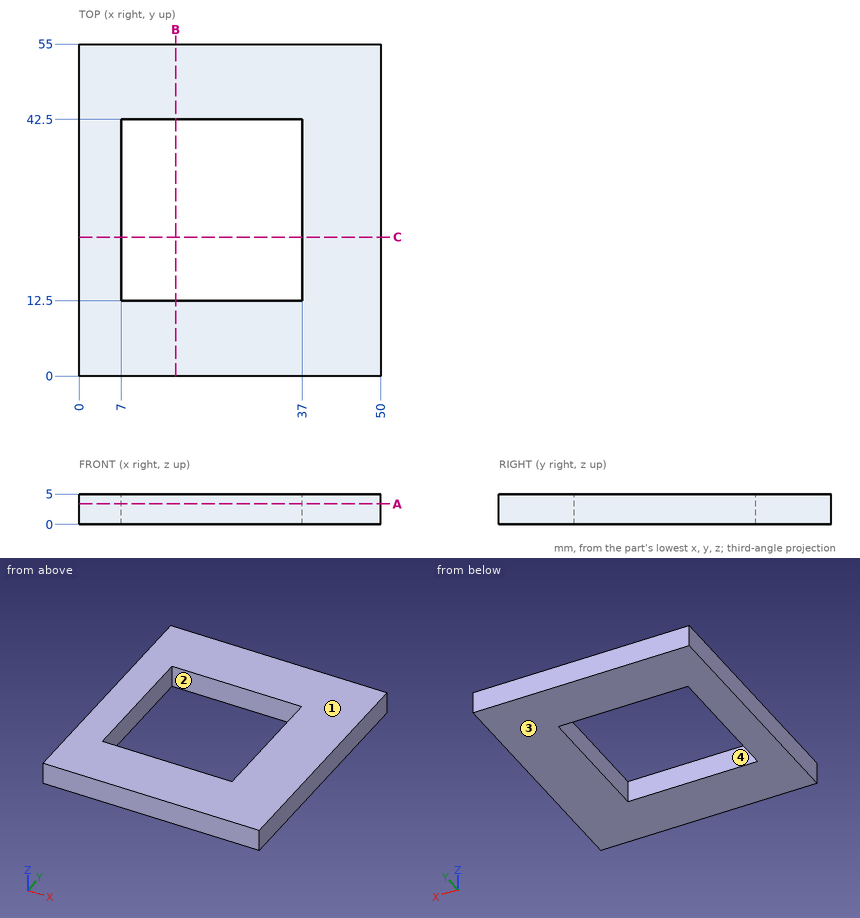
Drawing for the job (mm, zero at the part's lowest x, y, z). A direction names the side the tool comes from. Coordinates: 2 decimals unless noted, no trailing zeros. Order: outer loops, then holes, each group sorted by start corner. A loop starts at its lowest first (then second) coordinate and runs counter-clockwise, first axis right, second up. Notation, with made-up numbers: (17, 89) -> (31, 89) arc R34 cw to (31, 120) -> close; hole circle Ø7 at (-21.75, 23.5). An arc over 180 degrees is marked (long way). One line per item, written item: value.
(1) Slice it at B-B, the plane x = 16. List the corners of the cut face in (y, z), plus the area to 3 significant figures.
Checked values:
outline: (0, 0) -> (12.5, 0) -> (12.5, 5) -> (0, 5) -> close; (42.5, 0) -> (55, 0) -> (55, 5) -> (42.5, 5) -> close
area: 125 mm2
(2) Probe line 1 (X direction, y = 27, z = 0.5); line 2 (Y direction, x = 19.5, z = 2.7). List the from-to ranges inside material, lowest first. Write a range as [from, to].
Checked values:
line 1: [0, 7], [37, 50]
line 2: [0, 12.5], [42.5, 55]
(3) Slice it at A-A, the plane z = 3.4. List the corners of the cut face in (x, y), plus the area to 3 significant figures.
Checked values:
outline: (0, 0) -> (50, 0) -> (50, 55) -> (0, 55) -> close; hole (7, 12.5) -> (37, 12.5) -> (37, 42.5) -> (7, 42.5) -> close
area: 1,850 mm2
(4) Slice it at C-C, the plane y = 23. List the corners of the cut face in (x, z).
Checked values:
outline: (0, 0) -> (7, 0) -> (7, 5) -> (0, 5) -> close; (37, 0) -> (50, 0) -> (50, 5) -> (37, 5) -> close
(5) Mould opens along X. For the marked faces 1 and 2 say: pulls with the +X half, pulls with the -X half, needs draft (parallel to the pull), parting line crosses it, or undercut.
Checked values:
face 1: needs draft
face 2: undercut
(6) Tool access for the marked faces 3 and 4: list every direction of +Z, -Z, +X, -X, +Y, -Y with a clear straight run to the whole face (end or side of a thin tool).
Checked values:
face 3: -Z, +X, -X, +Y, -Y
face 4: +Z, -Z
